Source: three-view drawing plus pictorial views. Frame: mm from the lowest corner of the part. A direction names the side the tool comes from. Give positions to 0.01 mm unless a question says otherwise; leave off trailing zeros. Write each loop counter-clockwise with the first axis right and the second up, starting at its lowest first coordinate (ties: lowest second). Pieces come first, ordered by that corner, then holes.
Q1. Cut plane A-A on x = 5. Return the cut outline in (y, z).
Q2. Line query: L1, parallel to Y at x = 3.25, z = 1.25; L2, parallel to X at y = 1.25, z = 4.5; L3, parallel to Z at x = 8, y = 7.25. Output: solid intervals per line, ascending.
Q3. Cut plane D-D on z = 1. Return the cut outline in (x, y).
Q4. Reachability of the marked faces 1 and 2 from +Z, -Z, +X, -X, +Y, -Y: full face, straight path, thin tool, end or side. Return the list, or none.
Q5. Pin query (flat end, axial travel): pin 1 (1.5 mm diameter, centred on x = 1, z = 8.5, fed in from +Y). Return the tip coordinate at first contact, or that it passes through.
Q6. Cut plane C-C on y = 1.5. Return the cut outline in (x, z).
Q7. Cut plane B-B on z = 5. Return the cut outline in (x, y), plus the area to 3 significant figures.
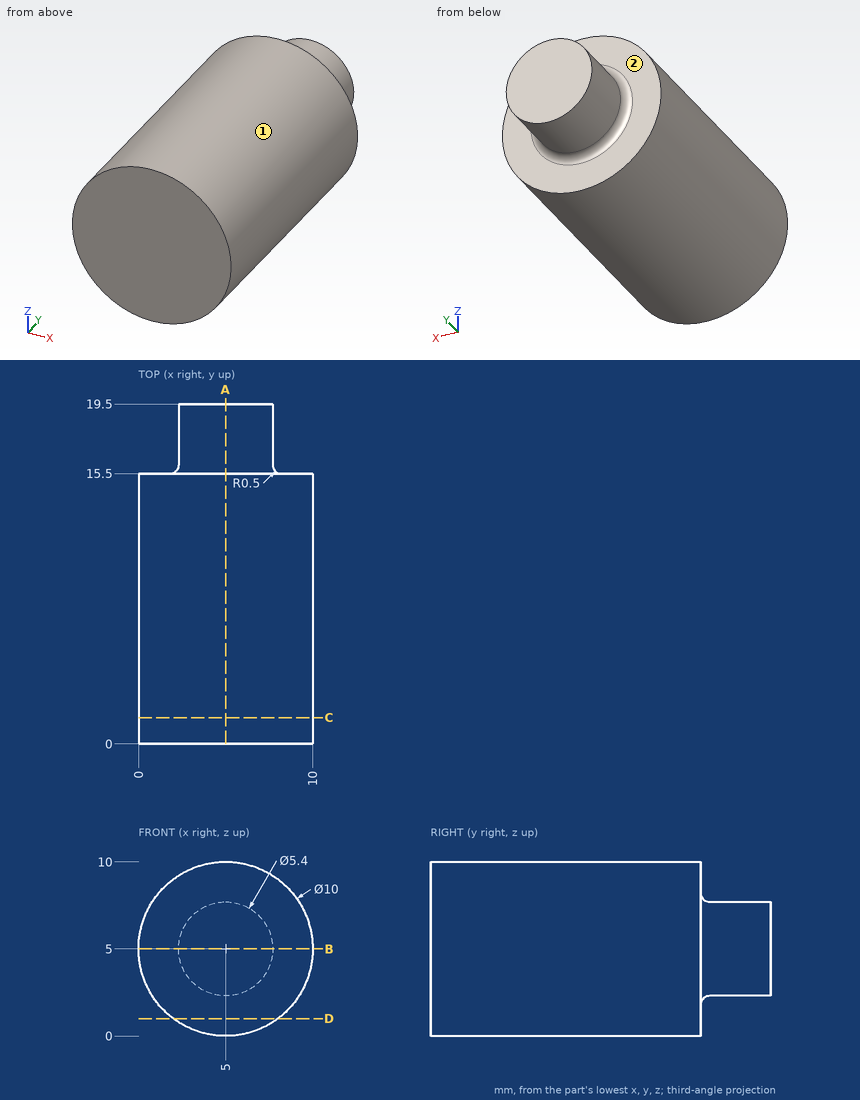
Data:
1. outline: (0, 0) - (15.5, 0) - (15.5, 1.8) arc R0.5 cw to (16, 2.3) - (19.5, 2.3) - (19.5, 7.7) - (16, 7.7) arc R0.5 cw to (15.5, 8.2) - (15.5, 10) - (0, 10) - close
2. L1: y = 0 to 15.5
2. L2: x = 0.03 to 9.97
2. L3: z = 1 to 9
3. outline: (2, 0) - (8, 0) - (8, 15.5) - (2, 15.5) - close
4. face 1: +Y, -Y
4. face 2: +Y
5. pin 1: stops at y = 15.5
6. outline: circle Ø10 at (5, 5)
7. outline: (0, 0) - (10, 0) - (10, 15.5) - (8.2, 15.5) arc R0.5 cw to (7.7, 16) - (7.7, 19.5) - (2.3, 19.5) - (2.3, 16) arc R0.5 cw to (1.8, 15.5) - (0, 15.5) - close
7. area: 177 mm2
